```python
from build123d import *

# Parameters (mm, degrees)
F0_R     = 1.5
F0_R_2   = 2.5
F1_DEPTH = 3


with BuildPart() as f1:
    # F0 (on Front) → F1 (new body)
    with BuildSketch(Plane.XZ):
        with BuildLine():
            ThreePointArc((-11.428203, -8.5), (-10.549524, -10.62132), (-8.428203, -11.5))
            Line((-8.428203, -11.5), (8.428203, -11.5))
            ThreePointArc((8.428203, -11.5), (10.549524, -10.62132), (11.428203, -8.5))
            Line((11.428203, -8.5), (11.428203, 8.5))
            ThreePointArc((11.428203, 8.5), (10.549524, 10.62132), (8.428203, 11.5))
            Line((8.428203, 11.5), (-8.428203, 11.5))
            ThreePointArc((-8.428203, 11.5), (-10.549524, 10.62132), (-11.428203, 8.5))
            Line((-11.428203, 8.5), (-11.428203, -8.5))
        make_face()
        with Locations((-6.928203, -7)):
            Circle(F0_R, mode=Mode.SUBTRACT)
        with Locations((6.928203, -7)):
            Circle(F0_R, mode=Mode.SUBTRACT)
        with Locations((-6.928203, 7)):
            Circle(F0_R, mode=Mode.SUBTRACT)
        with Locations((0, 6)):
            Circle(F0_R_2, mode=Mode.SUBTRACT)
        with Locations((6.928203, 7)):
            Circle(F0_R, mode=Mode.SUBTRACT)
    extrude(amount=F1_DEPTH)


solid = f1.part
```
Could you check a few things on this model? Use its own coordinates, in mm. Give positions to 0.01 mm unless a question says otherwise; leave off trailing zeros. Loops run counter-clockwise (first coordinate to the right, second up) from the corner with the lowest first, then second, coordinate; pieces in that order, holes last. Notation, with made-up numbers: (56.25, 33.25) - (87.25, 33.25) arc R11 ccw to (87.25, 41.25) - close; hole circle Ø10 at (-40, 41). An arc over 180 degrees is marked (long way). Use one line per item in the form item = value.
1. I want a section at C-C (x = 0). Please give me the cut outline in (y, z), and give its area (3 significant figures).
Response values:
outline = (-3, -11.5) - (0, -11.5) - (0, 3.5) - (-3, 3.5) - close; (-3, 8.5) - (0, 8.5) - (0, 11.5) - (-3, 11.5) - close
area = 54.0 mm²
2. I need wall thicknesses on probe 1 along X at (y, z) = (-1.95, 7.25); probe 2 along X at (y, z) = (-0.9, -8); probe 3 along Z at (x, y) = (8, -0.15). Which ranges of each line are inside material? Lowest first, please.
Response values:
probe_1 = -11.43 to -8.41, -5.45 to -2.17, 2.17 to 5.45, 8.41 to 11.43
probe_2 = -11.43 to -8.05, -5.81 to 5.81, 8.05 to 11.43
probe_3 = -11.5 to -8.05, -5.95 to 5.95, 8.05 to 11.5
3. I want a section at B-B (z = -7). Please give me the cut outline in (x, y).
Response values:
outline = (-11.43, -3) - (-8.43, -3) - (-8.43, 0) - (-11.43, 0) - close; (-5.43, -3) - (5.43, -3) - (5.43, 0) - (-5.43, 0) - close; (8.43, -3) - (11.43, -3) - (11.43, 0) - (8.43, 0) - close
4. Thinking about a two-plate mould opening in X: for faces 1 (the face through (-11.428, -1, 0)), 2 (the face through (10.57, -1.48, 10.6)), 3 (the face through (-0.33, -1.48, 8.48)), 4 (the face through (-8.12, -1.48, 6.09)), which applies, released by +X, released by -X, zero draft, split by the parting line, or undercut?
Response values:
face_1 = released by -X
face_2 = released by +X
face_3 = undercut
face_4 = undercut
5. I want a section at D-D (z = 7). Please give me the cut outline in (x, y).
Response values:
outline = (-11.43, -3) - (-8.43, -3) - (-8.43, 0) - (-11.43, 0) - close; (-5.43, -3) - (-2.29, -3) - (-2.29, 0) - (-5.43, 0) - close; (2.29, -3) - (5.43, -3) - (5.43, 0) - (2.29, 0) - close; (8.43, -3) - (11.43, -3) - (11.43, 0) - (8.43, 0) - close
6. I want a section at A-A (y = -2.55). Please give me the cut outline in (x, z).
Response values:
outline = (-11.43, -8.5) arc R3 ccw to (-8.43, -11.5) - (8.43, -11.5) arc R3 ccw to (11.43, -8.5) - (11.43, 8.5) arc R3 ccw to (8.43, 11.5) - (-8.43, 11.5) arc R3 ccw to (-11.43, 8.5) - close; hole circle Ø3 at (-6.93, -7); hole circle Ø3 at (-6.93, 7); hole circle Ø5 at (0, 6); hole circle Ø3 at (6.93, -7); hole circle Ø3 at (6.93, 7)
